Solid Edge part; units mm, degrees
sketch "Sketch1" plane through (0, 0, 0) normal (0, -1, 0) x (1, 0, 0)
  circle A0 centre (0, 0) radius 6
extrude "Protrusion1" add sketch "Sketch1" along normal mid plane 260
hole "Hole_1" at (0, -130, 0) direction (0, 1, 0) diameter 6.647 depth 10
hole "Hole_2" at (0, 130, 0) direction (0, -1, 0) diameter 6.647 depth 10
sketch "Sketch2" plane through (0, -75, 0) normal (0, -1, 0) x (1, 0, 0)
  line L0 (6, -6) -> (6, -10)
  line L1 (6, -10) -> (-124, -10)
  line L2 (-124, -10) -> (-124, -6)
  line L3 (-124, -6) -> (-6, -6)
  line L4 (-6, 0) -> (-6, -6)
  line L5 (6, 0) -> (6, -6)
  arc A0 (-6, 0) -> (6, 0) centre (0, 0) ccw
extrude "ExtrudedProtrusion_2" add sketch "Sketch2" along normal mid plane 40
fillet "Round_1" radius 5 2 edges at (-124, -95, -8) (-124, -55, -8)
hole "Hole_7" at (-111, -83, -6) direction (0, 0, -1) diameter 10 end up to next
hole "Hole1" at (-51, -83, -6) direction (0, 0, -1) diameter 10 end up to next
mirror "Mirror1" about plane through (0, 0, 0) normal (0, -1, 0) of "ExtrudedProtrusion_2", "Round_1", "Hole_7", "Hole1"
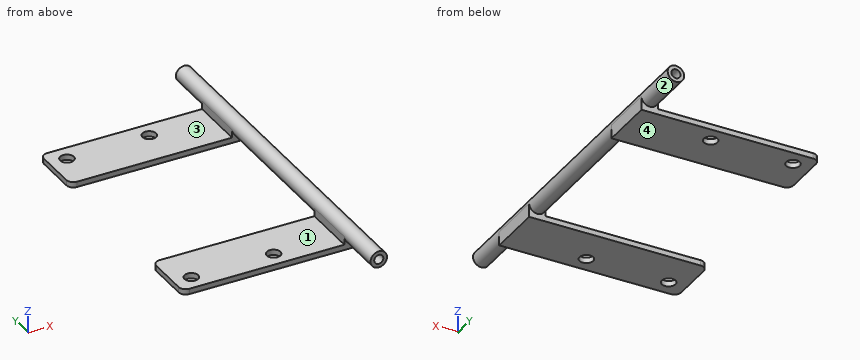
Verification items for the finished model (mm, model axes). Face numbers are marked on the shaded views. A direction names the side the tool comes from. Round coordinates to 2 decimals unless told otherwise and drop trailing zeros. Loops run counter-clockwise (first coordinate to the right, second up) from the corner with the lowest first, then second, coordinate; pieces in that order, holes last. Notation, with made-up numbers: (-31.75, 78) - (2.25, 78) arc R32 cw to (2.25, 110) - close; hole circle Ø2 at (-38.75, 45.25). An arc over 180 degrees is marked (long way). Answer in a Markdown table with one row per item. Add a question column.
Q1. Gauge pin test, flat ends, axial feed: pin 1 (1.8 mm diameter, centred on y = 82, z = -4, fed in from -X); pin 2 (9 mm diameter, centred on x = -51, y = 83, fed in from +Z); pin 3 (20 mm diameter, centred on x = -72, y = -79.5, fed in from +Z); pin 4 (3.5 mm diameter, centred on x = 0.5, z = -1, fed in from +Y). Record the tip position at first contact, or that the pin passes through.
Q2. Material ranges on line 1 (X direction, y = -83, z = -7.5); line 2 (Y direction, x = -51, z = -9.1); line 3 (Y direction, x = -37, z = -8.75), recorded low to high.
Q3. Tool access check on the marked faces 3 and 4. Record the directions out of +Z, -Z, +X, -X, +Y, -Y that give a thin tool (end or side, any length) a straight path to the whole face; none if there is none.
Q4. Section check A-A on y = 83. Enter the section's corners in (x, z).
Q5. Section check B-B on x = -51. Enter the section's corners in (y, z).
Q6. Section check D-D on y = -68.5. Enter the section's corners in (x, z), plus the area to 3 significant figures.
Q7. Release check for a two-part mould opening along Y. For the marked faces 1 and 2 record: pulls with the +Y half, pulls with the -Y half, needs draft (parallel to the pull), parting line crosses it, or undercut.
Q8. Section check C-C on x = -74. Enter the section's corners in (y, z), plus the area to 3 significant figures.
Found:
| question | item | result |
|---|---|---|
| 1 | pin 1 | stops at x = -6 |
| 1 | pin 2 | passes through |
| 1 | pin 3 | stops at z = -6 |
| 1 | pin 4 | stops at y = 120 |
| 2 | line 1 | x = -124 to -116, -106 to -56, -46 to 6 |
| 2 | line 2 | y = -95 to -88, -78 to -55, 55 to 78, 88 to 95 |
| 2 | line 3 | y = -95 to -55, 55 to 95 |
| 3 | face 3 | +Z, -X, +Y, -Y |
| 3 | face 4 | -Z, +X, -X, +Y, -Y |
| 4 | outline | (-124, -10) - (-116, -10) - (-116, -6) - (-124, -6) - close; (-106, -10) - (-56, -10) - (-56, -6) - (-106, -6) - close; (-46, -10) - (6, -10) - (6, 0) arc R6 ccw to (-6, 0) - (-6, -6) - (-46, -6) - close |
| 5 | outline | (-95, -10) - (-88, -10) - (-88, -6) - (-95, -6) - close; (-78, -10) - (-55, -10) - (-55, -6) - (-78, -6) - close; (55, -10) - (78, -10) - (78, -6) - (55, -6) - close; (88, -10) - (95, -10) - (95, -6) - (88, -6) - close |
| 6 | outline | (-124, -10) - (6, -10) - (6, 0) arc R6 ccw to (-6, 0) - (-6, -6) - (-124, -6) - close |
| 6 | area | 649 mm² |
| 7 | face 1 | needs draft |
| 7 | face 2 | undercut |
| 8 | outline | (-95, -10) - (-55, -10) - (-55, -6) - (-95, -6) - close; (55, -10) - (95, -10) - (95, -6) - (55, -6) - close |
| 8 | area | 320 mm² |
